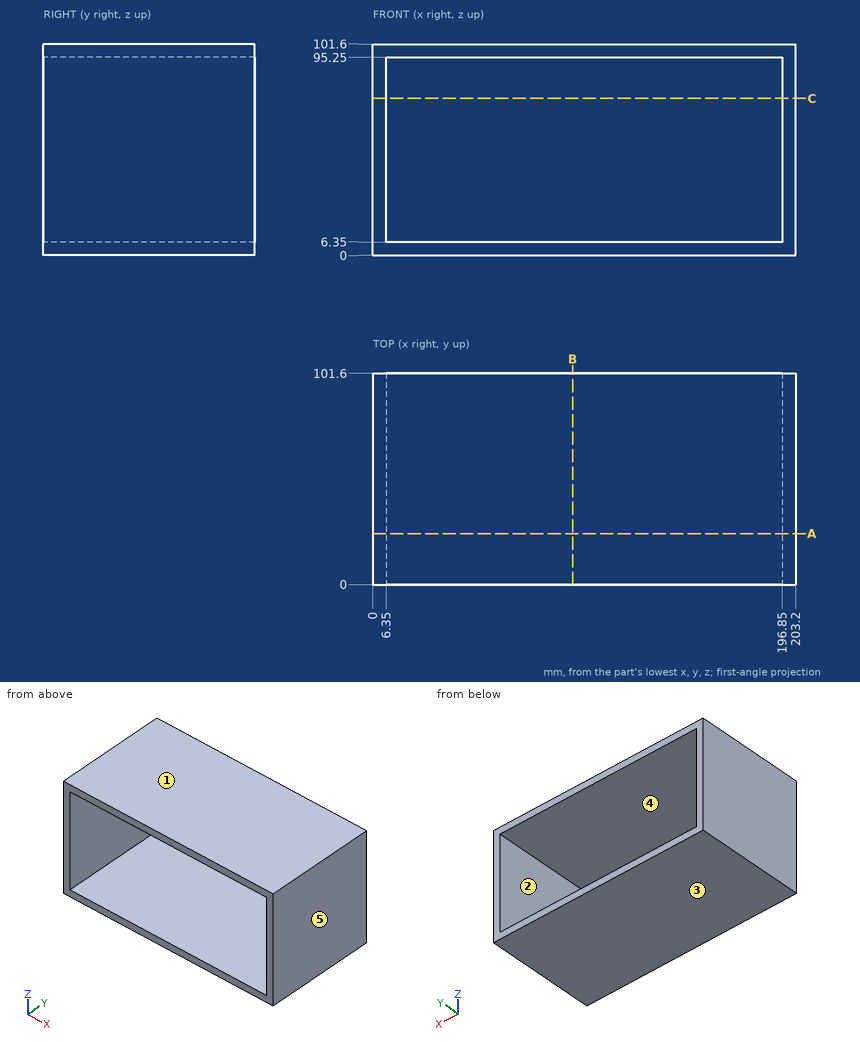
Answer from the drawing. Dimensions are ordinates in mm from the lowest x, y and z of the part. A direction names the side the tool comes from. Coordinates: 2 decimals unless noted, no trailing zeros. Write each loop counter-clockwise with the first axis right and the second up, starting at its lowest first coordinate (ties: lowest second). Pieces come first, ordered by that corner, then holes. Notation, with made-up numbers: M 3.25,-24 L 47.25,-24 A24 ccw 47.25,-4 Z; hole C -29.5,18 d4. An arc over 180 degrees is marked long. Write item = value, one per line.
1. The part is cut by section A-A (y = 24.5). Determine the outline of the cut face in (x, z), then the cut area to 3 significant figures.
Solution:
outline = M 0,0 L 203.2,0 L 203.2,101.6 L 0,101.6 Z; hole M 6.35,6.35 L 196.85,6.35 L 196.85,95.25 L 6.35,95.25 Z
area = 3,710 mm2
2. For the marked faces 4 and 5, determine the directions among +Z, -Z, +X, -X, +Y, -Y from which every point of the face is accessible in a straight line to the end or side of a thin tool.
Solution:
face_4 = +Y, -Y
face_5 = +Z, -Z, +X, +Y, -Y
3. Determine the mould class of the marked faces 1, 2 and 3 for opening direction Z: released by +Z, released by -Z, zero draft, split by the parting line, or undercut.
Solution:
face_1 = released by +Z
face_2 = undercut
face_3 = released by -Z
4. Straight lines are drawn through the part: line 1 (X direction, y = 72, z = 55); line 2 (Z direction, x = 77.5, y = 23). For each, find the intervals that lie inside material, in ascending order. Write a range as from..to.
Solution:
line_1 = 0..6.35, 196.85..203.2
line_2 = 0..6.35, 95.25..101.6
5. A flat-ended cylindrical pin translates along its axis: pin 1 (10 mm diameter, centred on x = 148, z = 14, fed in from +Y). Find the tip coordinate at first contact, or state that the pin passes through.
Solution:
pin_1 = through
6. The part is cut by section B-B (x = 96). Determine the outline of the cut face in (y, z).
Solution:
outline = M 0,0 L 101.6,0 L 101.6,6.35 L 0,6.35 Z; M 0,95.25 L 101.6,95.25 L 101.6,101.6 L 0,101.6 Z
7. The part is cut by section C-C (z = 75.5). Determine the outline of the cut face in (x, y), then the cut area to 3 significant figures.
Solution:
outline = M 0,0 L 6.35,0 L 6.35,101.6 L 0,101.6 Z; M 196.85,0 L 203.2,0 L 203.2,101.6 L 196.85,101.6 Z
area = 1,290 mm2
